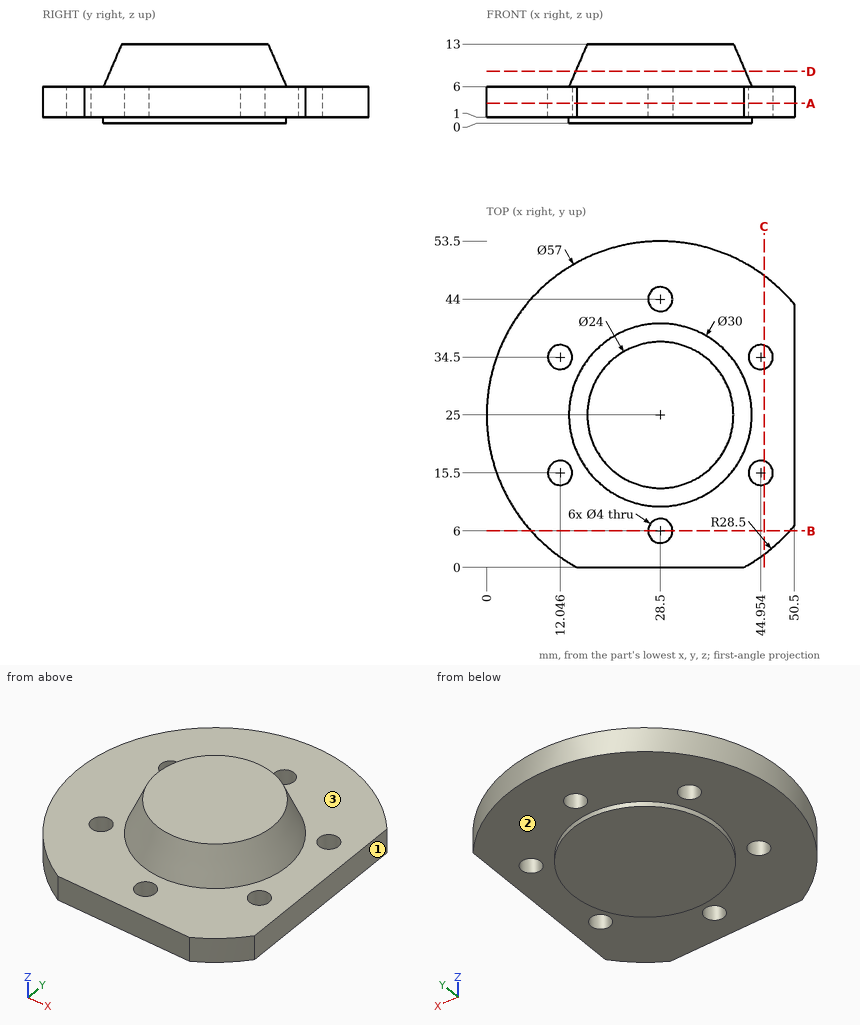
The figure shows three views and two pictorial views of one solid part (mm, origin at its lowest corner). Answer the questions. A direction names the side the tool comes from. Round coordinates to 2 decimals unless told otherwise and drop trailing zeros. Order: outer loops, then holes, each group sorted by start corner. A loop starts at its lowest first (then second) coordinate and runs counter-clockwise, first axis right, second up. Notation, with made-up numbers: M 33.25,33.25 L 87.25,33.25 A14 cw 87.25,54.25 Z; hole C 17.25,45 d3. An arc over 180 degrees is marked long. Put each result on its own line as item: value. Start each with the question number.
Q1. Flat-ended cylindrical pins translate along their axes: pin 1 (1 mm diameter, centred on y = 35.5, z = 7, fed in from +X); pin 2 (1.5 mm diameter, centred on x = 35, y = 47.5, fed in from -Z); pin 3 (3.5 mm diameter, centred on x = 44.95, y = 15.5, fed in from +Z); pin 4 (5 mm diameter, centred on x = 12.05, y = 15.5, fed in from +Z). Find the tip coordinate at first contact, or state that the pin passes through.
Q2. Straight lines are drawn through the part: L1, parallel to X at y = 34, z = 2.5; L2, parallel to Z at x = 23, y = 8; L3, parallel to X at y = 37, z = 2.25. For each, find the intervals that lie inside material, in ascending order. Write a range as [from, to].
Q3. Section A-A, the plane z = 3.25 is taken. Write down the section's boundary in (x, y) (1 decimal), and give its area (3 significant figures).
Q4. Section C-C, the plane x = 45.5 is taken. Write down the section's boundary in (y, z) (1 decimal), and give its area (3 significant figures).
Q5. A tool of negligible diameter and unlimited length cuts with its end or side. For the marked faces 1, 2 and 3, from which of +Z, -Z, +X, -X, +Y, -Y can it reach the whole face along a straight path? Write none if from no direction.
Q6. Section B-B, the plane y = 6 is taken. Write down the section's boundary in (x, z).
Q7. Section D-D, the plane z = 8.5 is taken. Write down the section's boundary in (x, y).
Findings below:
1. pin 1: stops at x = 39.18
1. pin 2: stops at z = 1
1. pin 3: passes through
1. pin 4: stops at z = 6
2. L1: x = [1.46, 10.11], [13.98, 43.02], [46.89, 50.5]
2. L2: z = [1, 6]
2. L3: x = [2.65, 50.5]
3. outline: M 14.8,0 L 42.2,0 A28.5 ccw 50.5,6.9 L 50.5,43.1 A28.5 ccw long Z; hole C 12,15.5 d4; hole C 12,34.5 d4; hole C 28.5,6 d4; hole C 28.5,44 d4; hole C 45,15.5 d4; hole C 45,34.5 d4
3. area: 2,250 mm^2
4. outline: M 2.1,1 L 13.6,1 L 13.6,6 L 2.1,6 Z; M 17.4,1 L 32.6,1 L 32.6,6 L 17.4,6 Z; M 36.4,1 L 47.9,1 L 47.9,6 L 36.4,6 Z
4. area: 190 mm^2
5. face 1: +Z, -Z, +X, +Y, -Y
5. face 2: -Z
5. face 3: +Z
6. outline: M 7.26,1 L 26.5,1 L 26.5,6 L 7.26,6 Z; M 30.5,1 L 49.74,1 L 49.74,6 L 30.5,6 Z
7. outline: C 28.5,25 d27.86
